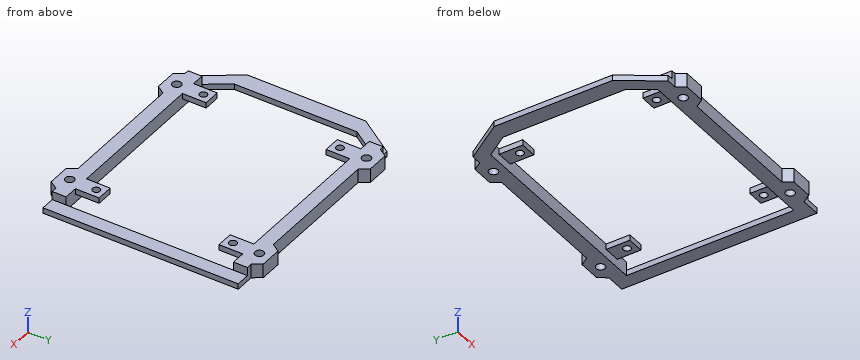
```python
from build123d import *

# Parameters (mm, degrees)
BODY_DEPTH                       = 5
SIDE_EXTRUSION_DEPTH             = 5
MOUNTING_HOLE_D                  = 3.2
MOUNTING_CUTOUT_REACH            = 80.058
SKETCH7_W                        = 3
SKETCH7_H                        = 8.5
SKETCH8_R                        = 1.35
MOUNTING_HOLE_CUTOUT_DEPTH       = 62.424750712
MOUNTING_MIRROR2_COPY_1_DEPTH    = 5
MOUNTING_MIRROR2_COPY_2_D        = 3.2
MOUNTING_MIRROR2_COPY_3_REACH    = 80.058
MOUNTING_MIRROR2_COPY_3_SKETCH_W = 3
MOUNTING_MIRROR2_COPY_3_SKETCH_H = 8.5
MOUNTING_MIRROR2_COPY_4_SKETCH_R = 1.35
MOUNTING_MIRROR2_COPY_4_DEPTH    = 62.424750712
SKETCH9_W                        = 5
SKETCH9_H                        = 70
SKETCH9_W_2                      = 11.445654338
RPI_SPACING_CUTOUT_DEPTH         = 3


with BuildPart() as part:
    # Sketch3 → body (new body)
    with BuildSketch(Plane.XY):
        Polygon((-48, 21.182653996), (-48, -21.182653996), (-38.594438725, -35), (42, -35), (42, 35), (-38.594438725, 35), align=None)
        Polygon((-26, 21.5), (-26, 30), (26, 30), (26, 21.5), (32, 21.5), (32, 30), (37, 30), (37, -30), (32, -30), (32, -21.5), (26, -21.5), (26, -30), (-26, -30), (-26, -21.5), (-32, -21.5), (-32, -30), (-36.554345662, -30), (-42, -22), (-42, 22), (-36.554345662, 30), (-32, 30), (-32, 21.5), align=None, mode=Mode.SUBTRACT)
    extrude(amount=BODY_DEPTH)

    # Sketch4 → side_extrusion (add)
    with BuildSketch(Plane.XY):
        Polygon((-35, 35), (-33, 38), (-25, 38), (-23, 35), align=None)
    side_extrusion = extrude(amount=SIDE_EXTRUSION_DEPTH)

    # mounting_hole (through all)
    with Locations(Plane.XY.offset(5)):
        with Locations((-29, 34)):
            mounting_hole = Hole(MOUNTING_HOLE_D / 2)

    # Sketch7 → mounting_cutout (cut, up to next)
    with BuildSketch(Plane(origin=(-26, 0, 0), x_dir=(0, 0, -1), z_dir=(1, 0, 0)), mode=Mode.PRIVATE) as mounting_cutout_sk1:
        with Locations((-1.5, 25.75)):
            Rectangle(SKETCH7_W, SKETCH7_H)
    mounting_cutout_tool1 = extrude(mounting_cutout_sk1.sketch, amount=-MOUNTING_CUTOUT_REACH, mode=Mode.PRIVATE) & part.part
    mounting_cutout = mounting_cutout_tool1.solids().sort_by_distance((-26, 25.75, 1.5))[0]
    add(mounting_cutout, mode=Mode.SUBTRACT)

    # Sketch8 → mounting_hole_cutout (cut, through all)
    with BuildSketch(Plane.XY.offset(5)):
        with Locations((-29, 24.5)):
            Circle(SKETCH8_R)
    mounting_hole_cutout = extrude(amount=-MOUNTING_HOLE_CUTOUT_DEPTH, mode=Mode.SUBTRACT)

    # mounting_mirror1: side_extrusion, mounting_hole, mounting_cutout, mounting_hole_cutout across plane
    add(side_extrusion.mirror(Plane(origin=(0, 0, 0), x_dir=(0, 0, 1), z_dir=(1, 0, 0))))
    add(mounting_hole.mirror(Plane(origin=(0, 0, 0), x_dir=(0, 0, 1), z_dir=(1, 0, 0))), mode=Mode.SUBTRACT)
    add(mounting_cutout.mirror(Plane(origin=(0, 0, 0), x_dir=(0, 0, 1), z_dir=(1, 0, 0))), mode=Mode.SUBTRACT)
    add(mounting_hole_cutout.mirror(Plane(origin=(0, 0, 0), x_dir=(0, 0, 1), z_dir=(1, 0, 0))), mode=Mode.SUBTRACT)

    # mounting_mirror2: side_extrusion, mounting_hole, mounting_cutout, mounting_hole_cutout across plane
    add(side_extrusion.mirror(Plane.ZX))
    add(mounting_hole.mirror(Plane.ZX), mode=Mode.SUBTRACT)
    add(mounting_cutout.mirror(Plane.ZX), mode=Mode.SUBTRACT)
    add(mounting_hole_cutout.mirror(Plane.ZX), mode=Mode.SUBTRACT)

    # mounting_mirror2 copy 1 sketch → mounting_mirror2 copy 1 (add)
    with BuildSketch(Plane(origin=(0, 0, 0), x_dir=(-1, 0, 0), z_dir=(0, 0, 1))):
        Polygon((-35, 35), (-33, 38), (-25, 38), (-23, 35), align=None)
    extrude(amount=MOUNTING_MIRROR2_COPY_1_DEPTH)

    # mounting_mirror2 copy 2 (through all)
    with Locations(Plane(origin=(0, 0, 5), x_dir=(-1, 0, 0), z_dir=(0, 0, 1))):
        with Locations((-29, 34)):
            Hole(MOUNTING_MIRROR2_COPY_2_D / 2)

    # mounting_mirror2 copy 3 sketch → mounting_mirror2 copy 3 (cut, up to next)
    with BuildSketch(Plane(origin=(26, 0, 0), x_dir=(0, 0, -1), z_dir=(-1, 0, 0)), mode=Mode.PRIVATE) as mounting_mirror2_copy_3_sk1:
        with Locations((-1.5, 25.75)):
            Rectangle(MOUNTING_MIRROR2_COPY_3_SKETCH_W, MOUNTING_MIRROR2_COPY_3_SKETCH_H)
    mounting_mirror2_copy_3_tool1 = extrude(mounting_mirror2_copy_3_sk1.sketch, amount=-MOUNTING_MIRROR2_COPY_3_REACH, mode=Mode.PRIVATE) & part.part
    add(mounting_mirror2_copy_3_tool1.solids().sort_by_distance((26, -25.75, 1.5))[0], mode=Mode.SUBTRACT)

    # mounting_mirror2 copy 4 sketch → mounting_mirror2 copy 4 (cut, through all)
    with BuildSketch(Plane(origin=(0, 0, 5), x_dir=(-1, 0, 0), z_dir=(0, 0, 1))):
        with Locations((-29, 24.5)):
            Circle(MOUNTING_MIRROR2_COPY_4_SKETCH_R)
    extrude(amount=-MOUNTING_MIRROR2_COPY_4_DEPTH, mode=Mode.SUBTRACT)

    # Sketch9 → rpi_spacing_cutout (cut)
    with BuildSketch(Plane.XY.offset(5)):
        with Locations((39.5, 0)):
            Rectangle(SKETCH9_W, SKETCH9_H)
        with Locations((-42.277172831, 0)):
            Rectangle(SKETCH9_W_2, SKETCH9_H)
    extrude(amount=-RPI_SPACING_CUTOUT_DEPTH, mode=Mode.SUBTRACT)


solid = part.part
```
CAD build for the part. Positions are in the model's coordinates, mm. Give positions to 0.01 mm unless a question says otherwise; leave off trailing zeros. Write each loop counter-clockwise with the first axis right and the second up, starting at its lowest first coordinate (ties: lowest second). Pieces come first, ordered by that corner, then holes. Notation, with made-up numbers: M 61,-28.5 L 103,-28.5 A15 ccw 103,-3.5 Z; hole C 6.25,24 d10. An arc over 180 degrees is marked long. Return JSON: item names as keys, results as strings. Group by question number.
(1) Flat gauge pins, fed straight in: pin 1 Ø1 at (y, z) = (24, 4.5) entering from -X; pin 2 Ø2.5 at (x, z) = (11, 3) entering from +Y; pin 3 Ø0.6 at (y, z) = (-27.5, 4.5) entering from +X. Where does each tip first touch, or does it go through?
(2) Drill centre lines: L1, parallel to Y at x = -29, z = 3.8; L2, parallel to Y at x = -29, z = 2.5; L3, parallel to Y at x = -16, z = 0.7. Where is each one in solid material? Low to high. Write a range as [from, to].
(3) Band-saw the part on A-A (x = -29). Give the cut face in (y, z).
(4) Band-saw the part on D-D (y = -34). Give the cut face in (x, z), and give its area (3 significant figures).
(5) Band-saw the part on B-B (y = -20). Give the cut face in (x, z), and give its area (3 significant figures).
(6) Band-saw the part on C-C (x = 2.5). Give the cut face in (y, z), and give its area (3 significant figures).
Entries:
{
 "1": {"pin 1": "stops at x = -32", "pin 2": "stops at y = 35", "pin 3": "stops at x = 32"},
 "2": {"L1": "y = [-38, -35.6], [-32.4, -25.85], [-23.15, -21.5], [21.5, 23.15], [25.85, 32.4], [35.6, 38]", "L2": "y = [-38, -35.6], [-32.4, -30], [30, 32.4], [35.6, 38]", "L3": "y = [-35, -30], [30, 35]"},
 "3": {"outline": "M -38,0 L -35.6,0 L -35.6,5 L -38,5 Z; M -32.4,0 L -30,0 L -30,3 L -25.85,3 L -25.85,5 L -32.4,5 Z; M -23.15,3 L -21.5,3 L -21.5,5 L -23.15,5 Z; M 21.5,3 L 23.15,3 L 23.15,5 L 21.5,5 Z; M 25.85,3 L 30,3 L 30,0 L 32.4,0 L 32.4,5 L 25.85,5 Z; M 35.6,0 L 38,0 L 38,5 L 35.6,5 Z"},
 "4": {"outline": "M -39.28,0 L -30.6,0 L -30.6,5 L -36.55,5 L -36.55,2 L -39.28,2 Z; M -27.4,0 L 27.4,0 L 27.4,5 L -27.4,5 Z; M 30.6,0 L 42,0 L 42,2 L 37,2 L 37,5 L 30.6,5 Z", "area": "351 mm^2"},
 "5": {"outline": "M -48,0 L -42,0 L -42,2 L -48,2 Z; M 37,0 L 42,0 L 42,2 L 37,2 Z", "area": "22.0 mm^2"},
 "6": {"outline": "M -35,0 L -30,0 L -30,5 L -35,5 Z; M 30,0 L 35,0 L 35,5 L 30,5 Z", "area": "50.0 mm^2"}
}
